Verification items for this drawing (mm, ordinates from the low corner). A direction names the side the tool comes from. Round coordinates to 2 decimals unless told otherwise and drop trailing zeros. Order: outer loops, then holes, each group sorted by start corner. A loop starts at its lowest first (then second) coordinate and runs counter-clockwise, first axis right, second up. Notation, with made-up numbers: (73, 35.5) -> (104, 35.5) arc R5 cw to (104, 42.5) -> close; hole circle Ø8 at (79.5, 26). An arc over 180 degrees is marked (long way). Use a Markdown table: item, result. Add a question column.
Item 1: Set-up check for the marked faces 1 and 2: record each of +Z, -Z, +X, -X, +Y, -Y from which the full face is reachable in a straight line by a thin tool's end or side.
Item 2: Sectioned sample at B-B, the plane x = 21.5. Record the cut outline in (y, z).
Item 3: Sectioned sample at D-D, the plane y = 56.5. Record the cut outline in (x, z).
Item 4: Gauge pin test, flat end, axial feed: pin 1 Ø1.5 at (x, y) = (28, 57) entering from +Z. Record the tip position at first contact, or that the pin passes through.
Item 5: Sectioned sample at C-C, the plane x = 28.5. Record the cut outline in (y, z).
Item 6: Material ranges on probe 1 along Y at (x, z) = (4, 32); probe 2 along Z at (x, y) = (33.5, 16), recorded low to high. Write a range as [from, to].
Item 7: Sectioned sample at A-A, the plane z = 17.5. Record the cut outline in (x, y), and give its area (3 significant figures).
Item 8: Mould release check, pull along Y, two halves, no side actions. Record for the marked faces 3, 4 and 5: pulls with the +Y half, pulls with the -Y half, needs draft (parallel to the pull), parting line crosses it, or undercut.
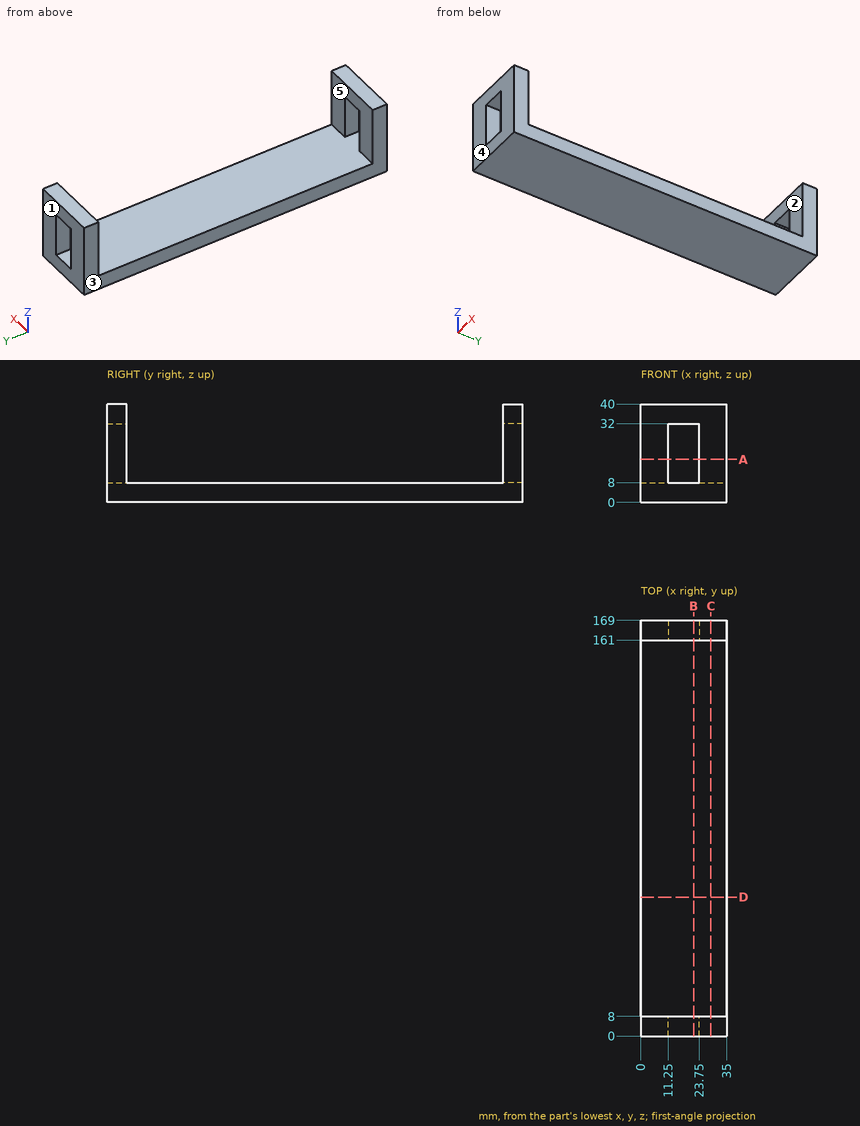
Found:
| question | item | result |
|---|---|---|
| 1 | face 1 | +Z, -Z, +X, -X, +Y |
| 1 | face 2 | +Z, +X, -X |
| 2 | outline | (0, 0) -> (169, 0) -> (169, 8) -> (0, 8) -> close; (0, 32) -> (8, 32) -> (8, 40) -> (0, 40) -> close; (161, 32) -> (169, 32) -> (169, 40) -> (161, 40) -> close |
| 3 | outline | (0, 0) -> (35, 0) -> (35, 8) -> (0, 8) -> close |
| 4 | pin 1 | stops at z = 8 |
| 5 | outline | (0, 0) -> (169, 0) -> (169, 40) -> (161, 40) -> (161, 8) -> (8, 8) -> (8, 40) -> (0, 40) -> close |
| 6 | probe 1 | y = [0, 8], [161, 169] |
| 6 | probe 2 | z = [0, 8] |
| 7 | outline | (0, 0) -> (11.25, 0) -> (11.25, 8) -> (0, 8) -> close; (0, 161) -> (11.25, 161) -> (11.25, 169) -> (0, 169) -> close; (23.75, 0) -> (35, 0) -> (35, 8) -> (23.75, 8) -> close; (23.75, 161) -> (35, 161) -> (35, 169) -> (23.75, 169) -> close |
| 7 | area | 360 mm2 |
| 8 | face 3 | needs draft |
| 8 | face 4 | pulls with the -Y half |
| 8 | face 5 | undercut |
